```python
from build123d import *

# Parameters (mm, degrees)
SKETCH1_W           = 200
SKETCH1_H           = 4.5
BOSS_EXTRUDE1_DEPTH = 4.5
SKETCH3_W           = 4.4
SKETCH3_H           = 75
CUT_EXTRUDE1_DEPTH  = 4.5
CUT_EXTRUDE2_REACH  = 6.5
SKETCH5_R           = 2.6


with BuildPart() as part:
    # Sketch1 → Boss-Extrude1 (new body)
    with BuildSketch(Plane(origin=(0, 0, 0), x_dir=(1, 0, 0), z_dir=(0, 1, 0))):
        Polygon((200, 75), (-200, 75), (-200, -75), (-100, -75), (-100, -70.5), (100, -70.5), (100, -75), (200, -75), align=None)
        with Locations((0, -77.25)):
            Rectangle(SKETCH1_W, SKETCH1_H)
        with Locations((0, -72.75)):
            Rectangle(SKETCH1_W, SKETCH1_H)
    extrude(amount=BOSS_EXTRUDE1_DEPTH)

    # Sketch3 → Cut-Extrude1 (cut)
    with BuildSketch(Plane(origin=(0, 4.5, 0), x_dir=(1, 0, 0), z_dir=(0, 1, 0))):
        with Locations((-147.8, 0)):
            Rectangle(SKETCH3_W, SKETCH3_H)
    cut_extrude1 = extrude(amount=-CUT_EXTRUDE1_DEPTH, mode=Mode.SUBTRACT)

    # Mirror1: Cut-Extrude1 across plane
    add(cut_extrude1.mirror(Plane(origin=(0, 0, 0), x_dir=(0, 0, 1), z_dir=(1, 0, 0))), mode=Mode.SUBTRACT)

    # Sketch5 → Cut-Extrude2 (cut, up to next)
    with BuildSketch(Plane(origin=(0, 4.5, 0), x_dir=(1, 0, 0), z_dir=(0, 1, 0)), mode=Mode.PRIVATE) as cut_extrude2_sk1:
        with Locations((-114.777861762, 45)):
            Circle(SKETCH5_R)
    cut_extrude2_tool1 = extrude(cut_extrude2_sk1.sketch, amount=-CUT_EXTRUDE2_REACH, mode=Mode.PRIVATE) & part.part
    add(cut_extrude2_tool1.solids().sort_by_distance((-114.777862, 4.5, -45))[0], mode=Mode.SUBTRACT)
    # Sketch5 → Cut-Extrude2 (cut, up to next)
    with BuildSketch(Plane(origin=(0, 4.5, 0), x_dir=(1, 0, 0), z_dir=(0, 1, 0)), mode=Mode.PRIVATE) as cut_extrude2_sk2:
        with Locations((170, 45)):
            Circle(SKETCH5_R)
    cut_extrude2_tool2 = extrude(cut_extrude2_sk2.sketch, amount=-CUT_EXTRUDE2_REACH, mode=Mode.PRIVATE) & part.part
    add(cut_extrude2_tool2.solids().sort_by_distance((170, 4.5, -45))[0], mode=Mode.SUBTRACT)
    # Sketch5 → Cut-Extrude2 (cut, up to next)
    with BuildSketch(Plane(origin=(0, 4.5, 0), x_dir=(1, 0, 0), z_dir=(0, 1, 0)), mode=Mode.PRIVATE) as cut_extrude2_sk3:
        with Locations((-134.777861762, 45)):
            Circle(SKETCH5_R)
    cut_extrude2_tool3 = extrude(cut_extrude2_sk3.sketch, amount=-CUT_EXTRUDE2_REACH, mode=Mode.PRIVATE) & part.part
    add(cut_extrude2_tool3.solids().sort_by_distance((-134.777862, 4.5, -45))[0], mode=Mode.SUBTRACT)
    # Sketch5 → Cut-Extrude2 (cut, up to next)
    with BuildSketch(Plane(origin=(0, 4.5, 0), x_dir=(1, 0, 0), z_dir=(0, 1, 0)), mode=Mode.PRIVATE) as cut_extrude2_sk4:
        with Locations((190, 45)):
            Circle(SKETCH5_R)
    cut_extrude2_tool4 = extrude(cut_extrude2_sk4.sketch, amount=-CUT_EXTRUDE2_REACH, mode=Mode.PRIVATE) & part.part
    add(cut_extrude2_tool4.solids().sort_by_distance((190, 4.5, -45))[0], mode=Mode.SUBTRACT)


solid = part.part
```
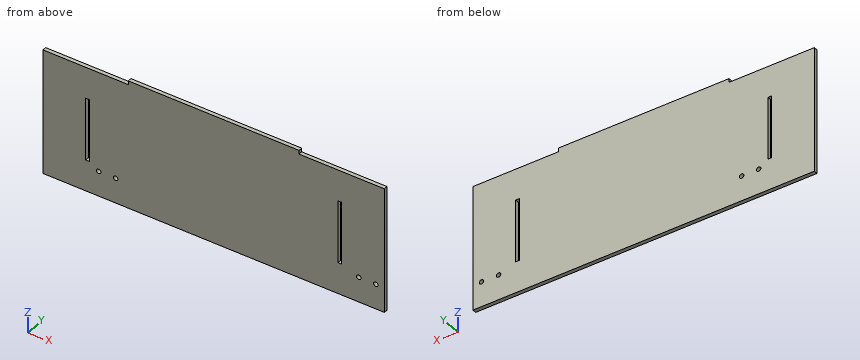
Here's how the part is built. I have some questions about the finished solid (model axes, mm). Round coordinates to 2 decimals unless told otherwise and drop trailing zeros. Write each loop counter-clockwise with the first axis right and the second up, starting at its lowest first coordinate (ties: lowest second). Pieces come first, ordered by that corner, then holes.
Q1. If we section it at C-C on x = -176: Write out the boundary of the cut face in (y, z), plus the area to 3 significant figures.
Q2. Will this pin go through, and if not, where does the flat tip stop? P1, Ø2, axis at x = -148, y = 2, coming from the +Z side.
Q3. Please list where these lines run through material, in increasing order: probe 1 along X at (y, z) = (0.8, -36); probe 2 along X at (y, z) = (2, -45); probe 3 along Z at (x, y) = (190, 1.75).
Q4. If we section it at B-B on z = 12.5: Write out the boundary of the cut face in (x, y), plus the area to 3 significant figures.
Q5. If we section it at A-A on y = 1.7: Write out the boundary of the cut face in (x, z).
Answer below:
1. outline: (0, -75) - (4.5, -75) - (4.5, 75) - (0, 75) - close
1. area: 675 mm2
2. P1: stops at z = 75
3. probe 1: x = -200 to -150, -145.6 to 145.6, 150 to 200
3. probe 2: x = -200 to -137.38, -132.18 to -117.38, -112.18 to 167.4, 172.6 to 187.4, 192.6 to 200
3. probe 3: z = -75 to -47.6, -42.4 to 75
4. outline: (-200, 0) - (-150, 0) - (-150, 4.5) - (-200, 4.5) - close; (-145.6, 0) - (145.6, 0) - (145.6, 4.5) - (-145.6, 4.5) - close; (150, 0) - (200, 0) - (200, 4.5) - (150, 4.5) - close
4. area: 1,760 mm2
5. outline: (-200, -75) - (200, -75) - (200, 75) - (100, 75) - (100, 79.5) - (-100, 79.5) - (-100, 75) - (-200, 75) - close; hole (-150, -37.5) - (-145.6, -37.5) - (-145.6, 37.5) - (-150, 37.5) - close; hole circle Ø5.2 at (-134.78, -45); hole circle Ø5.2 at (-114.78, -45); hole (145.6, -37.5) - (150, -37.5) - (150, 37.5) - (145.6, 37.5) - close; hole circle Ø5.2 at (170, -45); hole circle Ø5.2 at (190, -45)
